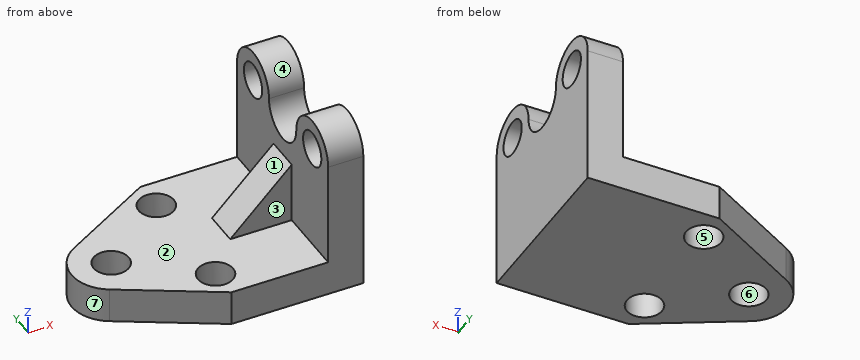
Autodesk Fusion 360 part; units mm, degrees
sketch "草图1" plane through (0, 0, 0) normal (0, 0, 1) x (1, 0, 0)
  line L0 (0, -40) -> (0, 55) construction
  line L1 (-75, 0) -> (190, 0) construction
  line L2 (0, -35) -> (0, -32.2208) construction
  line L3 (0, -20) -> (0, 20)
  line L4 (0, 20) -> (-22, 20)
  line L5 (-22, 20) -> (-43.4432, 7.8267)
  line L6 (0, -20) -> (-22, -20)
  line L7 (-22, -20) -> (-43.4432, -7.8267)
  arc A0 (-43.4432, 7.8267) -> (-43.4432, -7.8267) centre (-39, 0) ccw
  circle A1 centre (-39, 0) radius 4
  circle A2 centre (-22, 13) radius 4
  circle A3 centre (-22, -13) radius 4
  dimension "d1" = 40
  dimension "d2" = 22
  dimension "d3" = 39
  dimension "d4" = 9
  dimension "d5" = 8
  dimension "d6" = 26
  dimension "d7" = 22
extrude "拉伸1" add sketch "草图1" along normal blind 8
sketch "草图2" plane through (0, 0, 0) normal (1, 0, 0) x (0, 1, 0)
  line L0 (-20, 0) -> (20, 0)
  line L1 (20, 0) -> (20, 8)
  line L2 (20, 8) -> (-20, 8)
  line L3 (-20, 8) -> (-20, 0)
  line L4 (0, 39) -> (0, -13) construction
  line L5 (-35, 0) -> (42, 0) construction
  line L6 (-20, 0) -> (-20, 32)
  line L7 (20, 0) -> (20, 32)
  circle A0 centre (-13, 32) radius 4
  circle A1 centre (13, 32) radius 4
  arc A2 (-6, 32) -> (-20, 32) centre (-13, 32) ccw
  arc A3 (-6, 32) -> (6, 32) centre (0, 32) ccw
  arc A4 (20, 32) -> (6, 32) centre (13, 32) ccw
  dimension "d10" = 8
  dimension "d11" = 26
  dimension "d12" = 32
extrude "拉伸2" add sketch "草图2" along normal blind 8
sketch "草图3" plane through (0, 0, 0) normal (0, 1, 0) x (1, 0, 0)
  line L0 (0, -8) -> (-14, -8)
  line L1 (-14, -8) -> (0, -22)
  line L2 (0, -22) -> (0, -8)
  dimension "d15" = 14
  dimension "d16" = 14
extrude "拉伸3" add sketch "草图3" along normal mid plane 8
equation "d3 = 17 mm + 22 mm"
Input: part model. Units: mm. Frame: model coordinates. Face numbers are marked on the shaded views. A direction names the side the tool comes from. Give positions to 0.01 mm unless a question says otherwise; leave off trailing zeros. Order: outer loops, then holes, each group sorted by start corner. A loop starts at its lowest first (then second) coordinate and runs counter-clockwise, first axis right, second up.
Q1. Section C-C on y = 0. Output: boundary loops of the cut face in (x, z), and give its area (3 significant figures).
Checked values:
outline: (-48, 0) - (-43, 0) - (-43, 8) - (-48, 8) - close; (-35, 0) - (8, 0) - (8, 26) - (0, 26) - (0, 22) - (-14, 8) - (-35, 8) - close
area: 626 mm2
Q2. Contact query for flat-ended pins moving along their axis: pin 1 Ø12 at (x, y) = (-28.5, -6.5) entering from +Z; pin 2 Ø7 at (x, z) = (-9, 14) entering from -Y; pin 3 Ø7 at (x, z) = (-9, 12.5) entering from +Y; pin 4 Ø8 at (x, z) = (-41, 15) entering from -Y. Output: stop coordinate, or through.
Checked values:
pin 1: stops at z = 8
pin 2: stops at y = -4
pin 3: stops at y = 4
pin 4: passes through
Q3. Section D-D on x = -39. Output: boundary loops of the cut face in (y, z), and give its area (3 significant figures).
Checked values:
outline: (-10.35, 0) - (-4, 0) - (-4, 8) - (-10.35, 8) - close; (4, 0) - (10.35, 0) - (10.35, 8) - (4, 8) - close
area: 102 mm2
Q4. Ray query, probe 1 along Y at (x, z) = (-22, 2); probe 2 along Z at (x, y) = (4, -13); probe 3 along X at (y, z) = (-12, 20.5). Return the intervals inside material, ascending.
Checked values:
probe 1: y = -20 to -17, -9 to 9, 17 to 20
probe 2: z = 0 to 28, 36 to 39
probe 3: x = 0 to 8
Q5. Draft query along X for the marked faces 4, 5, 6 and 7. Return one class per face: +X half, -X half, draft (parallel to the pull), parting line (faces both ways), or undercut.
Checked values:
face 4: draft
face 5: undercut
face 6: undercut
face 7: -X half
Q6. Set-up query: the marked faces 1, 2 and 3. Return all of +Z, -Z, +X, -X, +Y, -Y with unobstructed straight access to the full face (end or side cutting, diameter ignored); none if empty.
Checked values:
face 1: +Z, -X, +Y, -Y
face 2: +Z, -X
face 3: +Z, -X, -Y
Q7. Section B-B on z = 12. Output: boundary loops of the cut face in (x, y), and give its area (3 significant figures).
Checked values:
outline: (-10, -4) - (0, -4) - (0, -20) - (8, -20) - (8, 20) - (0, 20) - (0, 4) - (-10, 4) - close
area: 400 mm2
Q8. Section A-A on y = -13. Output: boundary loops of the cut face in (x, z).
Checked values:
outline: (-34.33, 0) - (-26, 0) - (-26, 8) - (-34.33, 8) - close; (-18, 0) - (8, 0) - (8, 28) - (0, 28) - (0, 8) - (-18, 8) - close; (0, 36) - (8, 36) - (8, 39) - (0, 39) - close
